Here's the drawing with two shaded views (mm, measured from the low corner). I have some questions. Round coordinates to 2 decimals unless told otherwise and drop trailing zeros. Loops run counter-clockwise (first coordinate to the right, second up) from the corner with the lowest first, then second, coordinate; pieces in that order, holes last.
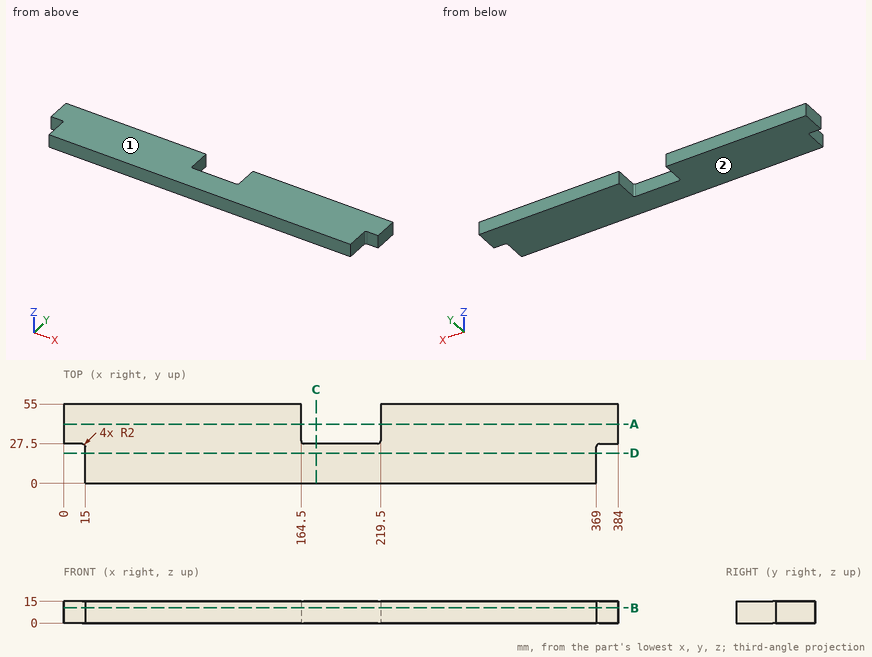
Item 1: Will these pins go through, and if not, where does the flat tip stop? pin 1 (1.5 mm diameter, centred on y = 23, z = 8, fed in from -X); pin 2 (3 mm diameter, centred on x = 116, y = 29, fed in from -Z); pin 3 (4 mm diameter, centred on x = 376.5, z = 10, fed in from -Y); pin 4 (4.5 mm diameter, centred on x = 203, z = 4.5, fed in from +Y).
Results list:
pin 1: stops at x = 15
pin 2: stops at z = 0
pin 3: stops at y = 27.5
pin 4: stops at y = 27.5
Item 2: If I drill on line 1 along X through (y, z) = (35, 7.75); line 2 along X through (y, z) = (29, 11.25); line 3 along X through (y, z) = (23, 6.25), over which ranges is the centre line in solid material (lowest first)?
Results list:
line 1: x = 0 to 164.5, 219.5 to 384
line 2: x = 0 to 164.56, 219.44 to 384
line 3: x = 15 to 369
Item 3: We'd pull the mould along Z, two halves only. Please class the marked faces 1 and 2: released by +Z, released by -Z, zero draft, split by the parting line, or undercut.
Results list:
face 1: released by +Z
face 2: released by -Z
Item 4: If we section it at D-D, the plane y = 21: Please give me the cut outline in (x, z).
Results list:
outline: (15, 0) - (369, 0) - (369, 15) - (15, 15) - close
Item 5: If we section it at C-C, the plane x = 175: Please give me the cut outline in (y, z).
Results list:
outline: (0, 0) - (27.5, 0) - (27.5, 15) - (0, 15) - close
Item 6: If we section it at A-A, the plane y = 41: Please give me the cut outline in (x, z), then the cut area to 4 significant figures.
Results list:
outline: (0, 0) - (164.5, 0) - (164.5, 15) - (0, 15) - close; (219.5, 0) - (384, 0) - (384, 15) - (219.5, 15) - close
area: 4,935 mm2
Item 7: If we section it at B-B, the plane z = 10.5: Please give me the cut outline in (x, y), then the cut area to 3 significant figures.
Results list:
outline: (0, 27.5) - (13, 27.5) arc R2 cw to (15, 25.5) - (15, 0) - (369, 0) - (369, 25.5) arc R2 cw to (371, 27.5) - (384, 27.5) - (384, 55) - (219.5, 55) - (219.5, 29.5) arc R2 cw to (217.5, 27.5) - (166.5, 27.5) arc R2 cw to (164.5, 29.5) - (164.5, 55) - (0, 55) - close
area: 18,800 mm2
